Could you check a few things on this model? Use its own coordinates, in mm. A direction names the side the tool comes from. Give positions to 0.01 mm unless a question says otherwise; leave off trailing zeros. Write each loop counter-clockwise with the first axis right and the second up, starting at its lowest first coordinate (ties: lowest second). Pieces come first, ordered by that corner, then holes. Notation, with made-up numbers: (2.25, 41) - (26.25, 41) arc R22 ccw to (26.25, 74) - close; hole circle Ø6 at (38, 75.5). An arc over 180 degrees is marked (long way). Use one line per item in the form item = value.
Autodesk Inventor part; units mm, degrees
ref_plane "YZ Plane" through (0, 0, 0) normal (1, 0, 0) x (0, 1, 0)
ref_plane "XZ Plane" through (0, 0, 0) normal (0, 1, 0) x (-1, 0, 0)
ref_plane "XY Plane" through (0, 0, 0) normal (0, 0, 1) x (1, 0, 0)
sketch "Sketch1" plane through (0, 0, 0) normal (0, 1, 0) x (-1, 0, 0)
  circle A0 centre (0, 0) radius 2
  dimension "d0" = 4
extrude "Extrusion1" add sketch "Sketch1" along normal blind 40
sketch "Sketch2" plane through (0, 40, 0) normal (0, 1, 0) x (1, 0, 0)
  circle A0 centre (0, 0) radius 3.5
  dimension "d3" = 7
extrude "Extrusion2" add sketch "Sketch2" along normal blind 3
sketch "Sketch3" plane through (0, 43, 0) normal (0, 1, 0) x (1, 0, 0)
  circle A0 centre (0, 0) radius 2
  line L0 (0, 2) -> (1.7321, 1)
  line L1 (1.7321, 1) -> (1.7321, -1)
  line L2 (1.7321, -1) -> (0, -2)
  line L3 (0, -2) -> (-1.7321, -1)
  line L4 (-1.7321, -1) -> (-1.7321, 1)
  line L5 (-1.7321, 1) -> (0, 2)
extrude "Extrusion3" cut sketch "Sketch3" against normal blind 2 contours L1 L2 L3 L4 L5 L0
properties part number "M4_hinge_bolt"
1. If we mould it in two halves opening along X, with no side actions, what happens to faces 1 (the face through (3.233, 41.479, -1.341)), 2 (the face through (2, 40, 2)), 3 (the face through (0.88, 42.01, 1.49))? For each: pulls with the +X half, pulls with the -X half, needs draft (parallel to the pull), parting line crosses it, or undercut.
Response values:
face_1 = parting line crosses it
face_2 = needs draft
face_3 = undercut
2. Which directions (+Z, -Z, +X, -X, +Y, -Y) give clear straight access to the entire face, cutting with the end or side of a thin tool? Please do faces 4 (the face through (1, 43, -2)), 5 (the face through (0, 20, 2)), 6 (the face through (-1.732, 42, 0)).
Response values:
face_4 = +Z, -Z, +X, -X, +Y
face_5 = -Y
face_6 = +Y
3. If I drill on line 1 (Y direction, x = -0.5, z = 3); line 2 (X direction, y = 6, z = -1); line 3 (Y direction, x = 0, z = 1.25), over which ranges is the centre line in solid material (lowest first)? Write a range as from..to.
Response values:
line_1 = 40..43
line_2 = -1.73..1.73
line_3 = 0..41
4. Imagine slicing it at A-A, the plane z = 0. List the corners of the cut face in (x, y) for me, and give its area (3 significant figures).
Response values:
outline = (-3.5, 40) - (-2, 40) - (-2, 0) - (2, 0) - (2, 40) - (3.5, 40) - (3.5, 43) - (1.73, 43) - (1.73, 41) - (-1.73, 41) - (-1.73, 43) - (-3.5, 43) - close
area = 174 mm²
5. For pin 1 (3 mm diameter, centred on x = -0.5, y = 19, fed in from +Z); pin 2 (1.5 mm diameter, centred on y = 24, z = -2, fed in from +X); pin 3 (2 mm diameter, centred on x = -2.5, y = 23, fed in from -Z), each with a flat end and sliding along its axis, tell me the tip position at first contact or that it passes through.
Response values:
pin_1 = 2
pin_2 = 1.56
pin_3 = -1.32
6. Imagine slicing it at C-C, the plane y = 19.5. List the corners of the cut face in (x, z) for me, and give its area (3 significant figures).
Response values:
outline = circle Ø4 at (0, 0)
area = 12.6 mm²
7. Imagine slicing it at D-D, the plane x = -3. List the corners of the cut face in (y, z) for me.
Response values:
outline = (40, -1.8) - (43, -1.8) - (43, 1.8) - (40, 1.8) - close
8. Imagine slicing it at B-B, the plane x = -0.75. List the corners of the cut face in (y, z) for me.
Response values:
outline = (0, -1.85) - (40, -1.85) - (40, -3.42) - (43, -3.42) - (43, -1.57) - (41, -1.57) - (41, 1.57) - (43, 1.57) - (43, 3.42) - (40, 3.42) - (40, 1.85) - (0, 1.85) - close
